Can you work these out from the model? Positions are in its coordinate system, mm. A direction names the side the tool comes from. Coordinates: 2 decimals unless noted, no trailing zeros. Order: outer loops, then holes, each group sorted by start corner. A loop starts at its lowest first (then second) coordinate and runs counter-clockwise, first axis right, second up. Notation, with made-up numbers: (28.5, -9) -> (53.5, -9) arc R23 ccw to (53.5, 17) -> close; hole circle Ø6 at (83, 50.5). An arc over 180 degrees is marked (long way). Answer in a Markdown table with one row per item.
```python
from build123d import *

# Parameters (mm, degrees)
SKETCH_1_W                       = 41
SKETCH_1_H                       = 44
SM_BASE_FLANGE_1_DEPTH           = 3
SM_EDGE_FLANGE_1_STRIP_W         = 17
SM_EDGE_FLANGE_1_STRIP_H         = 3
SM_EDGE_FLANGE_1_STRIP_CUT_DEPTH = 44
SM_EDGE_FLANGE_1_DEPTH           = 44
SKETCH_11_R                      = 16
CUT_EXTRUDE_1_DEPTH              = 10
HOLE_WIZARD_M3_1_D               = 3.1
HOLE_WIZARD_M3_1_DEPTH           = 5.2
HOLE_WIZARD_M3_1_CSINK_D         = 6.4
HOLE_WIZARD_M3_1_CSINK_ANGLE     = 90
HOLE_WIZARD_M3_1_TIP             = 0.931333959
CUT_EXTRUDE_START                = -10
CUT_EXTRUDE_2_DEPTH              = 10
HOLE_WIZARD_M2_5_1_D             = 2.7
HOLE_WIZARD_M2_5_1_DEPTH         = 5.2
HOLE_WIZARD_M2_5_1_CSINK_D       = 5.6
HOLE_WIZARD_M2_5_1_CSINK_ANGLE   = 90
HOLE_WIZARD_M2_5_1_TIP           = 0.811161836
SM_EDGE_FLANGE_2_STRIP_W         = 17
SM_EDGE_FLANGE_2_STRIP_H         = 3
SM_EDGE_FLANGE_2_STRIP_CUT_DEPTH = 44
SM_EDGE_FLANGE_2_DEPTH           = 44
FILLET_1_R                       = 4
FILLET_2_R                       = 1
HOLE_WIZARD_M3_2_AT_2_COUNT      = 2
HOLE_WIZARD_M3_2_AT_2_PITCH      = 7.430637089
HOLE_WIZARD_M3_2_AT_3_COUNT      = 2
HOLE_WIZARD_M3_2_AT_3_PITCH      = 27.919799484
HOLE_WIZARD_M3_2_AT_4_COUNT      = 2
HOLE_WIZARD_M3_2_AT_4_PITCH      = 33.587572106
SKETCH_28_R                      = 18
CUT_EXTRUDE_3_DEPTH              = 10
SKETCH_29_R                      = 7.5
CUT_EXTRUDE_4_DEPTH              = 10
SKETCH_30_W                      = 10
SKETCH_30_H                      = 14
CUT_EXTRUDE_5_DEPTH              = 9
CUT_EXTRUDE_6_DEPTH              = 10
FILLET_3_R                       = 2
FILLET_4_R                       = 5
FILLET_5_R                       = 1


# Sheet-metal steps are written as plain solids
with BuildPart() as part:
    # Sketch 1 → 基体-法兰1 (new body)
    with BuildSketch(Plane(origin=(0, 0, 0), x_dir=(1, 0, 0), z_dir=(0, 1, 0))):
        Rectangle(SKETCH_1_W, SKETCH_1_H)
    extrude(amount=-SM_BASE_FLANGE_1_DEPTH)

    # 边线-法兰1 strip (across the edge) → 边线-法兰1 strip cut (cut)
    with BuildSketch(Plane(origin=(-20.5, 0, -22), x_dir=(1, 0, 0), z_dir=(0, 0, 1))):
        with Locations((-6, -1.5)):
            Rectangle(SM_EDGE_FLANGE_1_STRIP_W, SM_EDGE_FLANGE_1_STRIP_H)
    extrude(amount=SM_EDGE_FLANGE_1_STRIP_CUT_DEPTH, mode=Mode.SUBTRACT)

    # 边线-法兰1 section (across the edge) → 边线-法兰1 (add)
    with BuildSketch(Plane(origin=(-20.5, 0, -22), x_dir=(1, 0, 0), z_dir=(0, 0, 1))):
        with BuildLine():
            Line((-3, 2.5), (-3, 55))
            Line((-3, 55), (0, 55))
            Line((0, 55), (0, 2.5))
            ThreePointArc((0, 2.5), (0.732233047, 0.732233047), (2.5, 0))
            Line((2.5, 0), (2.5, -3))
            ThreePointArc((2.5, -3), (-1.389087297, -1.389087297), (-3, 2.5))
        make_face()
    extrude(amount=SM_EDGE_FLANGE_1_DEPTH)

    # 草图11 → 切除-拉伸1 (cut)
    with BuildSketch(Plane(origin=(-20.5, 0, 0), x_dir=(0, 0, -1), z_dir=(1, 0, 0))):
        with Locations(Location((0, 32, 0), (0, 0, 90))):
            Circle(SKETCH_11_R)
    extrude(amount=-CUT_EXTRUDE_1_DEPTH, mode=Mode.SUBTRACT)

    # M3 开槽半沉头螺钉的锥形沉头孔1
    with Locations(Plane(origin=(0, 0, 0), x_dir=(1, 0, 0), z_dir=(0, 1, 0))):
        with Locations((0, 12), (10.392304845, -6), (-10.392304845, -6)):
            CounterSinkHole(HOLE_WIZARD_M3_1_D / 2, HOLE_WIZARD_M3_1_CSINK_D / 2, depth=HOLE_WIZARD_M3_1_DEPTH, counter_sink_angle=HOLE_WIZARD_M3_1_CSINK_ANGLE)
            with Locations((0, 0, -(HOLE_WIZARD_M3_1_DEPTH + HOLE_WIZARD_M3_1_TIP / 2))):  # 118° drill point
                Cone(0, HOLE_WIZARD_M3_1_D / 2, HOLE_WIZARD_M3_1_TIP, mode=Mode.SUBTRACT)

    # 草图17 → 切除-拉伸2 (cut)
    with BuildSketch(Plane.ZY.offset(23.5).offset(CUT_EXTRUDE_START)):
        with BuildLine():
            Line((-16, 32), (-16, 55))
            ThreePointArc((-16, 55), (0, 71), (16, 55))
            Line((16, 55), (16, 32))
            ThreePointArc((16, 32), (0, 16), (-16, 32))
        make_face()
    extrude(amount=CUT_EXTRUDE_2_DEPTH, mode=Mode.SUBTRACT)

    # M2.5 开槽半沉头螺钉的锥形沉头孔1
    with Locations(Plane.ZY.offset(23.5)):
        with Locations((19.214153616, 18.040100258), (19.214153616, 45.959899742), (-19.214153616, 45.959899742), (-19.214153616, 18.040100258), (-13.959899742, 12.785846384), (13.959899742, 12.785846384)):
            CounterSinkHole(HOLE_WIZARD_M2_5_1_D / 2, HOLE_WIZARD_M2_5_1_CSINK_D / 2, depth=HOLE_WIZARD_M2_5_1_DEPTH, counter_sink_angle=HOLE_WIZARD_M2_5_1_CSINK_ANGLE)
            with Locations((0, 0, -(HOLE_WIZARD_M2_5_1_DEPTH + HOLE_WIZARD_M2_5_1_TIP / 2))):  # 118° drill point
                Cone(0, HOLE_WIZARD_M2_5_1_D / 2, HOLE_WIZARD_M2_5_1_TIP, mode=Mode.SUBTRACT)

    # 边线-法兰2 strip (across the edge) → 边线-法兰2 strip cut (cut)
    with BuildSketch(Plane(origin=(20.5, 0, 22), x_dir=(-1, 0, 0), z_dir=(0, 0, -1))):
        with Locations((-6, -1.5)):
            Rectangle(SM_EDGE_FLANGE_2_STRIP_W, SM_EDGE_FLANGE_2_STRIP_H)
    extrude(amount=SM_EDGE_FLANGE_2_STRIP_CUT_DEPTH, mode=Mode.SUBTRACT)

    # 边线-法兰2 section (across the edge) → 边线-法兰2 (add)
    with BuildSketch(Plane(origin=(20.5, 0, 22), x_dir=(-1, 0, 0), z_dir=(0, 0, -1))):
        with BuildLine():
            Line((-3, 2.5), (-3, 25))
            Line((-3, 25), (0, 25))
            Line((0, 25), (0, 2.5))
            ThreePointArc((0, 2.5), (0.732233047, 0.732233047), (2.5, 0))
            Line((2.5, 0), (2.5, -3))
            ThreePointArc((2.5, -3), (-1.389087297, -1.389087297), (-3, 2.5))
        make_face()
    extrude(amount=SM_EDGE_FLANGE_2_DEPTH)

    # 圆角1
    fillet_1_edges = [part.edges().sort_by_distance(p)[0] for p in [
        (22, 25, 22),
        (22, 25, -22),
        (-22, 55, -22),
        (-22, 55, 22),
    ]]
    fillet(fillet_1_edges, radius=FILLET_1_R)

    # 圆角2
    fillet_2_edges = [part.edges().sort_by_distance(p)[0] for p in [
        (-22, 55, -16),
        (-22, 55, 16),
    ]]
    fillet(fillet_2_edges, radius=FILLET_2_R)

    # 草图27 → M3 开槽半沉头螺钉的锥形沉头孔2 (revolve, cut)
    with BuildSketch(Plane(origin=(23.5, 12.785846384, 13.959899742), x_dir=(0, 0, -1), z_dir=(0, 1, 0))):
        Polygon((0, 0), (0, 3), (1.7, 3), (1.7, 1.5), (3.2, 0), align=None)
    hole_wizard_m3_2 = revolve(axis=Axis((29.85, 12.785846384, 13.959899742), (-1, 0, 0)), mode=Mode.SUBTRACT)

    # M3 开槽半沉头螺钉的锥形沉头孔2 at 2: M3 开槽半沉头螺钉的锥形沉头孔2 ×2
    with Locations(*[Vector(2.6296433264448836e-15, 0.7071067811865475, 0.7071067811865477) * (i * HOLE_WIZARD_M3_2_AT_2_PITCH) for i in range(1, HOLE_WIZARD_M3_2_AT_2_COUNT)]):
        add(hole_wizard_m3_2, mode=Mode.SUBTRACT)

    # M3 开槽半沉头螺钉的锥形沉头孔2 at 3: M3 开槽半沉头螺钉的锥形沉头孔2 ×2
    with Locations(*[(0, 0, -i * HOLE_WIZARD_M3_2_AT_3_PITCH) for i in range(1, HOLE_WIZARD_M3_2_AT_3_COUNT)]):
        add(hole_wizard_m3_2, mode=Mode.SUBTRACT)

    # M3 开槽半沉头螺钉的锥形沉头孔2 at 4: M3 开槽半沉头螺钉的锥形沉头孔2 ×2
    with Locations(*[Vector(0, 0.15643446504022762, -0.9876883405951383) * (i * HOLE_WIZARD_M3_2_AT_4_PITCH) for i in range(1, HOLE_WIZARD_M3_2_AT_4_COUNT)]):
        add(hole_wizard_m3_2, mode=Mode.SUBTRACT)

    # 草图28 → 切除-拉伸3 (cut)
    with BuildSketch(Plane(origin=(23.5, 0, 0), x_dir=(0, 0, -1), z_dir=(1, 0, 0))):
        with Locations((0, 32)):
            Circle(SKETCH_28_R)
    extrude(amount=-CUT_EXTRUDE_3_DEPTH, mode=Mode.SUBTRACT)

    # 草图29 → 切除-拉伸4 (cut)
    with BuildSketch(Plane.XZ.offset(3)):
        with Locations(Location((0, 0, 0), (0, 0, 270))):
            Circle(SKETCH_29_R)
    extrude(amount=-CUT_EXTRUDE_4_DEPTH, mode=Mode.SUBTRACT)

    # 草图30 → 切除-拉伸5 (cut)
    with BuildSketch(Plane.XZ.offset(3)):
        with Locations((-21, 0)):
            Rectangle(SKETCH_30_W, SKETCH_30_H)
    extrude(amount=-CUT_EXTRUDE_5_DEPTH, mode=Mode.SUBTRACT)

    # 草图32 → 切除-拉伸6 (cut)
    with BuildSketch(Plane.ZY.offset(23.5)):
        Polygon((-22, 22.040100258), (-13.879481118, 24.040100258), (-13.879481118, 65.768696361), (-22, 65.768696361), align=None)
        Polygon((13.879481118, 65.768696361), (13.879481118, 24.040100258), (22, 22.040100258), (22, 65.768696361), align=None)
    extrude(amount=-CUT_EXTRUDE_6_DEPTH, mode=Mode.SUBTRACT)

    # 圆角3
    fillet_3_edges = [part.edges().sort_by_distance(p)[0] for p in [
        (-22, 22.040100258, -22),
        (-22, 22.040100258, 22),
    ]]
    fillet(fillet_3_edges, radius=FILLET_3_R)

    # 圆角4
    fillet_4_edges = [part.edges().sort_by_distance(p)[0] for p in [
        (-22, 24.040100258, 13.879481118),
        (-22, 24.040100258, -13.879481118),
    ]]
    fillet(fillet_4_edges, radius=FILLET_4_R)

    # 圆角5
    fillet_5_edges = [part.edges().sort_by_distance(p)[0] for p in [
        (-22, 6, -7),
        (-16, -1.5, -7),
        (-22, 6, 7),
        (-16, -1.5, 7),
    ]]
    fillet(fillet_5_edges, radius=FILLET_5_R)


solid = part.part
```
(1) Suppose I cut it at B-B (z = 0). Please give me the cut outline in (x, y).
Response values:
| item | result |
|---|---|
| outline | (-23.5, 6) -> (-20.5, 6) -> (-20.5, 16) -> (-23.5, 16) -> close; (-16, -3) -> (-7.5, -3) -> (-7.5, 0) -> (-16, 0) -> close; (7.5, -3) -> (18, -3) arc R5.5 ccw to (23.5, 2.5) -> (23.5, 14) -> (20.5, 14) -> (20.5, 2.5) arc R2.5 cw to (18, 0) -> (7.5, 0) -> close |
(2) Suppose I cut it at A-A (y = 3.75). Please give me the cut outline in (x, z), and give its area (3 significant figures).
Response values:
| item | result |
|---|---|
| outline | (-23.5, -22) -> (-20.5, -22) -> (-20.5, -7) -> (-23.5, -7) -> close; (-23.5, 7) -> (-20.5, 7) -> (-20.5, 22) -> (-23.5, 22) -> close; (20.5, -22) -> (23.5, -22) -> (23.5, 22) -> (20.5, 22) -> close |
| area | 222 mm2 |
(3) We'd pull the mould along X, two halves only. Please class faces 1 (the flat face through (23.5, 11, 0)), 2 (the cylindrical face through (-20, 1, 14)), 3 (the flat face through (0, -1, -22)): +X half, -X half, draft (parallel to the pull), parting line (faces both ways), or undercut.
Response values:
| item | result |
|---|---|
| face 1 | +X half |
| face 2 | undercut |
| face 3 | draft |
(4) I need wall thicknesses on line 1 (X direction, y = 11.5, z = -20); line 2 (X direction, y = 23.5, z = 17); line 3 (Y direction, x = -8.5, z = 19.5). Which ranges of each line are inside material? Lowest first, please. Write a range as [from, to].
Response values:
| item | result |
|---|---|
| line 1 | [-23.5, -20.5], [20.5, 23.5] |
| line 2 | [20.5, 23.5] |
| line 3 | [-3, 0] |
(5) Will these pins go through, and if not, where does the flat tip stop? pin 1 Ø2 at (y, z) = (18.04, -19.21) entering from +X; pin 2 Ø1.5 at (y, z) = (-1.5, -1) entering from -X; pin 3 Ø3.5 at (y, z) = (18.04, -19.21) entering from -X; pin 4 Ø5 at (x, z) = (-12.5, 10) entering from +Y.
Response values:
| item | result |
|---|---|
| pin 1 | through |
| pin 2 | x = -16 |
| pin 3 | x = -22.45 |
| pin 4 | y = 0 |
(6) On a 3-axis mill with a long thin cutter (end or side, diameter ignored), from which of +Z, -Z, +X, -X, +Y, -Y can I reach the whole of each face in a straight line? I mean faces 4 (the cylindrical face through (-21.979, 23.145, 14.483)), 5 (the flat face through (-22.021, 22.816, -18.85)), 6 (the flat face through (-16, -2, 0)). Say none if no direction works.
Response values:
| item | result |
|---|---|
| face 4 | -X, +Y |
| face 5 | -Z, -X, +Y |
| face 6 | -X, +Y, -Y |
(7) Suppose I cut it at D-D (x = 16.5). Please give me the cut outline in (y, z).
Response values:
| item | result |
|---|---|
| outline | (-3, -22) -> (0, -22) -> (0, 22) -> (-3, 22) -> close |
(8) Suppose I cut it at C-C (x = 4). Please give me the cut outline in (y, z).
Response values:
| item | result |
|---|---|
| outline | (-3, -22) -> (0, -22) -> (0, -6.34) -> (-3, -6.34) -> close; (-3, 6.34) -> (0, 6.34) -> (0, 22) -> (-3, 22) -> close |
